CAD build for the part. Positions are in the model's coordinates, mm. A direction names the side the tool comes from. Round coordinates to 2 decimals unless told otherwise and drop trailing zeros. Write each loop counter-clockwise with the first axis right and the second up, starting at its lowest first coordinate (ties: lowest second). Pieces come first, ordered by that corner, then holes. Notation, with made-up numbers: (30, -19) - (60, -19) arc R22 ccw to (60, -11) - close; hole circle Ø11 at (57, 4). An arc over 180 degrees is marked (long way). Use one line per item in the form item = value. Start each with the question number.
Item 1: Pull direction X, two halves, no side cores. Call faces 3 (the cylindrical face through (204.544, 1.521, 17.013)), 4 (the flat face through (61, 3, 6)), 5 (the cylindrical face through (190.014, 1.521, 6.354)): +X half, -X half, draft (parallel to the pull), parting line (faces both ways), or undercut.
Item 2: Pin check, flat tips, straight feed: pin 1 (4 mm diameter, centred on x = 0, z = 15.5, fed in from -Y); pin 2 (0.9 mm diameter, centred on x = 153, y = 1.5, fed in from -Z). Stop position of each tip, or through.
Item 3: Band-saw the part on A-A, the plane y = 2.05. List the corners of the cut face in (x, z).
Item 4: Drill centre lines: L1, parallel to Z at x = 0, y = 1.95; L2, parallel to Z at x = -15.5, y = 0.7; L3, parallel to X at y = 1.65, z = 15.5. Where is each one in solid material? Low to high.
Item 5: Tool access for faces 1 (the flat face through (69.747, 1.479, -10.607)), 2 (the flat face through (97.872, 1.479, 25.298)): list every direction of +Z, -Z, +X, -X, +Y, -Y with a clear straight run to the whole face (end or side of a thin tool).
Item 6: Band-saw the part on B-B, the plane z = 24. List the corners of the cut face in (x, y).
Item 7: Band-saw the part on C-C, the plane x = 26. List the corners of the cut face in (y, z), and give its area (3 significant figures).
from build123d import *

# Parameters (mm, degrees)
BOSS_EXTRUDE1_DEPTH            = 3
M3_CLEARANCE_HOLE1_D           = 3.2
M3_CLEARANCE_HOLE1_CSINK_D     = 3.25
M3_CLEARANCE_HOLE1_CSINK_ANGLE = 90
FILLET2_R                      = 11


with BuildPart() as part:
    # Sketch1 → Boss-Extrude1 (new body)
    with BuildSketch(Plane(origin=(0, 0, 0), x_dir=(1, 0, 0), z_dir=(0, 1, 0))):
        with BuildLine():
            ThreePointArc((8.529623766, 28.761876128), (-29.78438528, 3.590319411), (1.450480292, -29.964914599))
            Line((1.450480292, -29.964914599), (207.5, -19.990892525))
            Line((207.5, -19.990892525), (207.5, -7.5))
            ThreePointArc((207.5, -7.5), (200, 0), (192.5, -7.5))
            Line((192.5, -7.5), (130.80460541, -7.5))
            Line((130.80460541, -7.5), (8.529623766, 28.761876128))
        make_face()
    extrude(amount=BOSS_EXTRUDE1_DEPTH)

    # M3 Clearance Hole1 (through all)
    with Locations(Plane(origin=(0, 3, 0), x_dir=(1, 0, 0), z_dir=(0, 1, 0))):
        with Locations((-15.5, 0), (0, 15.5), (15.5, 0), (0, -15.5)):
            CounterSinkHole(M3_CLEARANCE_HOLE1_D / 2, M3_CLEARANCE_HOLE1_CSINK_D / 2, counter_sink_angle=M3_CLEARANCE_HOLE1_CSINK_ANGLE)

    # Fillet2
    fillet2_edges = [part.edges().sort_by_distance(p)[0] for p in [
        (130.80460541, 1.5, 7.5),
        (192.5, 1.5, 7.5),
        (207.5, 1.5, 19.990892525),
    ]]
    fillet(fillet2_edges, radius=FILLET2_R)


solid = part.part
Determined:
q1.face_3 = +X half
q1.face_4 = draft
q1.face_5 = undercut
q2.pin_1 = 0
q2.pin_2 = 7.5
q3.outline = (1.45, 29.96) arc R30 ccw (long way) to (8.53, -28.76) - (129.27, 7.05) arc R11 cw to (132.4, 7.5) - (185.13, 7.5) arc R11 cw to (193.97, 3.04) arc R7.5 ccw to (207.5, 7.5) - (207.5, 9.51) arc R11 ccw to (197.03, 20.5) - close; hole circle Ø3.2 at (-15.5, 0); hole circle Ø3.2 at (0, -15.5); hole circle Ø3.2 at (0, 15.5); hole circle Ø3.2 at (15.5, 0)
q4.L1 = -30 to -17.1, -13.9 to 13.9, 17.1 to 30
q4.L2 = -25.69 to -1.6, 1.6 to 25.69
q4.L3 = -25.69 to -1.6, 1.6 to 205.73
q5.face_1 = -Z, +Y, -Y
q5.face_2 = +Z, +X, +Y, -Y
q6.outline = (-18, 0) - (124.68, 0) - (124.68, 3) - (-18, 3) - close
q7.outline = (0, -23.58) - (3, -23.58) - (3, 28.78) - (0, 28.78) - close
q7.area = 157 mm²
